Autodesk Inventor part; units mm, degrees
ref_plane "YZ Plane" through (0, 0, 0) normal (1, 0, 0) x (0, 1, 0)
ref_plane "XZ Plane" through (0, 0, 0) normal (0, 1, 0) x (-1, 0, 0)
ref_plane "XY Plane" through (0, 0, 0) normal (0, 0, 1) x (1, 0, 0)
sketch "草圖1" plane through (0, 0, 0) normal (0, 1, 0) x (-1, 0, 0)
  line L0 (0, 0) -> (-40, 0)
  line L1 (-40, 0) -> (-40, -60)
  line L2 (-40, -60) -> (0, -60)
  line L3 (0, -60) -> (0, 0)
  line L4 (-10, -30) -> (-30, -30)
  line L5 (-30, -30) -> (-30, -10)
  line L6 (-30, -10) -> (-10, -10)
  line L7 (-10, -10) -> (-10, -30)
  dimension "d0" = 10
  dimension "d1" = 10
  dimension "d2" = 20
  dimension "d3" = 60
  dimension "d4" = 20
  dimension "d5" = 10
extrude "擠出1" add sketch "草圖1" along normal blind 20
sketch "草圖2" plane through (40, 0, -60) normal (0, 0, -1) x (-1, 0, 0)
  line L0 (0, 20) -> (40, 20)
  line L1 (40, 20) -> (0, 20)
  line L2 (0, 20) -> (0, 30)
  line L3 (0, 30) -> (10, 30)
  line L4 (10, 30) -> (30, 40)
  line L5 (30, 40) -> (40, 40)
  line L6 (40, 40) -> (40, 20)
  point P0 (40, 0)
  dimension "d8" = 10
  dimension "d9" = 10
  dimension "d10" = 20
  dimension "d11" = 20
extrude "擠出2" add sketch "草圖2" against normal blind 20
chamfer "倒角1" distance 20 angle 45 1 edges at (30, 10, -10)
fillet "圓角1" radius 20 1 edges at (40, 10, 0)
properties part number "37"
Design review of the part built by this model. Coordinates are the model's own, in mm. A direction names the side the tool comes from. Give positions to 0.01 mm unless a question says otherwise; leave off trailing zeros. Write each loop counter-clockwise with the first axis right and the second up, starting at its lowest first coordinate (ties: lowest second). Pieces come first, ordered by that corner, then holes. Notation, with made-up numbers: M 45,7 L 91,7 A33 cw 91,44 Z; hole C -15.5,70.25 d9. An arc over 180 degrees is marked long. Answer as a JSON object with one key per item and string values. Group by question number.
1) For line 1 along Y through (x, z) = (19, -4); line 2 along Y through (x, z) = (30.5, -51); line 3 along Z through (x, y) = (25, 19.5), list the stretches that pass through material, from the lowest coordinate up.
2) Clearance check with flat-ended pins moving along their axes: pin 1 Ø4 at (x, z) = (34.5, -46.5) entering from +Y; pin 2 Ø10 at (x, y) = (22.5, 26.5) entering from +Z; pin 3 Ø4 at (x, z) = (10, -14.5) entering from +Y. State where each tip first meets the part, or that it passes through.
3) Tool access review of faces 4 (the face through (16, 28, -40)), 5 (the face through (20, 10, -20)), 6 (the face through (5, 40, -50)), 7 (the face through (20, 15, -60)), 8 (the face through (35, 30, -50)): name each direction out of +Z, -Z, +X, -X, +Y, -Y from which nothing blocks a thin tool from reaching the whole face with its end or side.
4) We need section B-B (x = 28). Give the boundary of the cut face in (y, z).
5) We need section C-C (z = -27.5). Give the boundary of the cut face in (x, y), and give its area (3 significant figures).
6) Mouldability with a two-part tool opening along Z and no side actions: class faces 1 (the face through (33.986, 10.14, -5.703)), 2 (the face through (10, 10, -20)), 3 (the face through (40, 11, -40)) as released by +Z, released by -Z, zero draft, split by the parting line, or undercut.
7) We need section D-D (z = -55). Give the boundary of the cut face in (x, y).
Answer key:
{
 "1": {"line 1": "y = 0 to 20", "line 2": "y = 0 to 30", "line 3": "z = -60 to -30, -25 to -0.64"},
 "2": {"pin 1": "stops at y = 30", "pin 2": "stops at z = -40", "pin 3": "stops at y = 20"},
 "3": {"face 4": "+Z, +X, -X, +Y", "face 5": "+Y, -Y", "face 6": "+Z, -Z, +X, -X, +Y", "face 7": "-Z, +X, -X, +Y, -Y", "face 8": "+Z, -Z, +X, +Y"},
 "4": {"outline": "M 0,-60 L 31,-60 L 31,-40 L 20,-40 L 20,-30 L 0,-30 Z; M 0,-28 L 20,-28 L 20,-1.67 L 0,-1.67 Z"},
 "5": {"outline": "M 0,0 L 10,0 L 10,20 L 0,20 Z; M 27.5,0 L 40,0 L 40,20 L 27.5,20 Z", "area": "450 mm²"},
 "6": {"face 1": "released by +Z", "face 2": "undercut", "face 3": "zero draft"},
 "7": {"outline": "M 0,0 L 40,0 L 40,30 L 30,30 L 10,40 L 0,40 Z"}
}
